```python
from build123d import *

# Parameters (mm, degrees)
ESQUISSE1_W             = 12
ESQUISSE1_H             = 60
MAIN_DEPTH              = 49.95
ESQUISSE2_R             = 1.25
HOLESFIXFORLCD_DEPTH    = 13
SKETCH1_W               = 98
SKETCH1_H               = 40.5
LCDWINDOWHOLE_DEPTH     = 13
SKETCH6_W               = 2.9
SKETCH6_H               = 2
MAKERBEAMRAIL_DEPTH     = 60
SKETCH7_W               = 50
SKETCH7_H               = 9.75
LCDPINSHOLES_DEPTH      = 6
SKETCH8_W               = 8
SKETCH8_H               = 40.5
REINFORCEMENT_DEPTH     = 2.5
REINFORCEMENT_2_DEPTH   = 2.5
SKETCH12_W              = 2.5
SKETCH12_H              = 69
WINDOWPLASTICHOLE_DEPTH = 104.9
SKETCH13_W              = 2.9
SKETCH13_H              = 1
MAKERBEAMRAILUP_DEPTH   = 103.9
BOSS_EXTRUDE2_DEPTH     = 12
SKETCH15_R              = 1.5
CUT_EXTRUDE4_DEPTH      = 7
BOSS_EXTRUDE3_DEPTH     = 10
SKETCH17_R              = 1.5
CUT_EXTRUDE5_DEPTH      = 114.9


with BuildPart() as part:
    # Esquisse1 → Main (new body, symmetric)
    with BuildSketch(Plane.XY):
        with Locations((6, 30)):
            Rectangle(ESQUISSE1_W, ESQUISSE1_H)
    extrude(amount=MAIN_DEPTH, both=True)

    # Esquisse2 → HolesFixForLCD (cut, through all)
    with BuildSketch(Plane(origin=(12, 0, 0), x_dir=(0, 0, -1), z_dir=(1, 0, 0))):
        with Locations((46.4, 2.5)):
            Circle(ESQUISSE2_R)
        with Locations((-46.4, 2.5)):
            Circle(ESQUISSE2_R)
        with Locations((46.4, 57.1)):
            Circle(ESQUISSE2_R)
        with Locations((-46.4, 57.1)):
            Circle(ESQUISSE2_R)
    extrude(amount=-HOLESFIXFORLCD_DEPTH, mode=Mode.SUBTRACT)

    # Sketch1 → LCDWindowHole (cut, through all)
    with BuildSketch(Plane(origin=(12, 0, 0), x_dir=(0, 0, -1), z_dir=(1, 0, 0))):
        with Locations((0, 30)):
            Rectangle(SKETCH1_W, SKETCH1_H)
    extrude(amount=-LCDWINDOWHOLE_DEPTH, mode=Mode.SUBTRACT)

    # Sketch6 → MakerBeamRail (add)
    with BuildSketch(Plane(origin=(0, 60, 0), x_dir=(1, 0, 0), z_dir=(0, 1, 0))):
        with Locations((5, 50.95)):
            Rectangle(SKETCH6_W, SKETCH6_H)
        with Locations((5, -50.95)):
            Rectangle(SKETCH6_W, SKETCH6_H)
    extrude(amount=-MAKERBEAMRAIL_DEPTH)

    # Sketch7 → LCDPinsHoles (cut)
    with BuildSketch(Plane(origin=(12, 0, 0), x_dir=(0, 0, -1), z_dir=(1, 0, 0))):
        with Locations((16.95, 55.125)):
            Rectangle(SKETCH7_W, SKETCH7_H)
    extrude(amount=-LCDPINSHOLES_DEPTH, mode=Mode.SUBTRACT)


with BuildPart() as body_2:
    # Sketch8 → Reinforcement (new body)
    with BuildSketch(Plane.ZY):
        with Locations((-45, 30)):
            Rectangle(SKETCH8_W, SKETCH8_H)
    extrude(amount=-REINFORCEMENT_DEPTH)


with BuildPart() as body_3:
    # Sketch8 → Reinforcement 2 (new body)
    with BuildSketch(Plane.ZY):
        with Locations((45, 30)):
            Rectangle(SKETCH8_W, SKETCH8_H)
    extrude(amount=-REINFORCEMENT_2_DEPTH)


with BuildPart() as windowplastichole_tool:
    # Sketch12 → WindowPlasticHole (new body, through all)
    with BuildSketch(Plane.XY.offset(51.95)):
        with Locations((1.25, 34.5)):
            Rectangle(SKETCH12_W, SKETCH12_H)
    extrude(amount=-WINDOWPLASTICHOLE_DEPTH)


with BuildPart() as part_1:
    add(part.part)

    # WindowPlasticHole: cut by windowplastichole_tool
    add(windowplastichole_tool.part, mode=Mode.SUBTRACT)

    # Sketch13 → MakerBeamRailUp (add)
    with BuildSketch(Plane.XY.offset(51.95)):
        with Locations((5, 60.5)):
            Rectangle(SKETCH13_W, SKETCH13_H)
    extrude(amount=-MAKERBEAMRAILUP_DEPTH)

    # Sketch14 → Boss-Extrude2 (add)
    with BuildSketch(Plane(origin=(0, 0, -49.95), x_dir=(-1, 0, 0), z_dir=(0, 0, -1))):
        Polygon((-12, 60), (-6.45, 60), (-6.45, 61), (-2.5, 61), (-2.5, 55), (-12, 55), align=None)
    extrude(amount=BOSS_EXTRUDE2_DEPTH)

    # Sketch15 → Cut-Extrude4 (cut, through all)
    with BuildSketch(Plane.XZ.offset(-55)):
        with Locations((5, -56.95)):
            Circle(SKETCH15_R)
    extrude(amount=-CUT_EXTRUDE4_DEPTH, mode=Mode.SUBTRACT)

    # Sketch16 → Boss-Extrude3 (add)
    with BuildSketch(Plane(origin=(0, 0, 0), x_dir=(-1, 0, 0), z_dir=(0, -1, 0))):
        Polygon((-2.5, -49.95), (-3.55, -49.95), (-3.55, -51.95), (-10, -51.95), (-10, -41.95), (-2.5, -41.95), align=None)
    extrude(amount=BOSS_EXTRUDE3_DEPTH)

    # Sketch17 → Cut-Extrude5 (cut, through all)
    with BuildSketch(Plane.XY.offset(51.95)):
        with Locations((5, -5)):
            Circle(SKETCH17_R)
    extrude(amount=-CUT_EXTRUDE5_DEPTH, mode=Mode.SUBTRACT)


with BuildPart() as body_2_1:
    add(body_2.part)

    # WindowPlasticHole: cut by windowplastichole_tool
    add(windowplastichole_tool.part, mode=Mode.SUBTRACT)


with BuildPart() as body_3_1:
    add(body_3.part)

    # WindowPlasticHole: cut by windowplastichole_tool
    add(windowplastichole_tool.part, mode=Mode.SUBTRACT)


solid = part_1.part
```
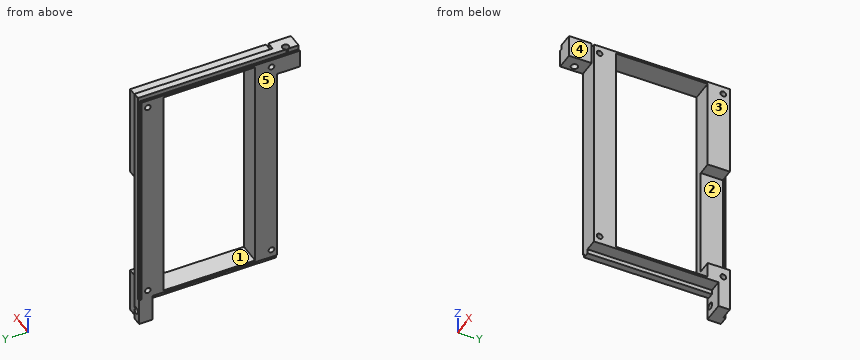
Check sheet for the modelled part. Datum: model origin and axes. Units: mm. Face numbers are marked on the shaded views. A direction names the side the tool comes from. Coordinates: 2 decimals unless noted, no trailing zeros. Loops run counter-clockwise (first coordinate to the right, second up) from the corner with the lowest first, then second, coordinate; pieces in that order, holes last.
1) Sectioned sample at A-A (y = 57.1). Record the boundary of the cut face in (x, z).
2) Material ranges on probe 1 along Y at (x, z) = (6.5, -46.4); probe 2 along Y at (x, z) = (5.25, 46.4); probe 3 along Y at (x, z) = (3.5, -17), recorded low to high.
3) Access from +Z, -Z, +X, -X, +Y, -Y to the whole of each face (thin tool, end or side, straight path). Record for the marked faces 4 and 5.
4) Gauge pin test, flat ends, axial feed: pin 1 (1 mm diameter, centred on x = 9, y = 24.5, fed in from +Z); pin 2 (3 mm diameter, centred on x = 8.5, y = 33.5, fed in from -Z); pin 3 (5 mm diameter, centred on y = 55, z = -6, fed in from +X). Record the tip position at first contact, or that the pin passes through.
5) Sectioned sample at B-B (z = 22.5). Record the boundary of the cut face in (x, y), and give its area (3 significant figures).
6) Sectioned sample at C-C (y = 48.5). Record the boundary of the cut face in (x, z), and give its area (4 significant figures).
7) Sectioned sample at D-D (z = 46.4). Record the boundary of the cut face in (x, y), and give its area (3 significant figures).
8) Release check for a two-part mould opening along Y. For the marked faces 1, 2 and 3 record: released by +Y, released by -Y, zero draft, split by the parting line, or undercut.
Check sheet entries:
1. outline: (2.5, -61.95) - (12, -61.95) - (12, -47.65) - (2.5, -47.65) - close; (2.5, -45.15) - (12, -45.15) - (12, -41.95) - (6, -41.95) - (6, 8.05) - (12, 8.05) - (12, 45.15) - (2.5, 45.15) - close; (2.5, 47.65) - (12, 47.65) - (12, 49.95) - (6.45, 49.95) - (6.45, 51.95) - (3.55, 51.95) - (3.55, 49.95) - (2.5, 49.95) - close; hole circle Ø3 at (5, -56.95)
2. probe 1: y = 0 to 1.25, 3.75 to 9.75, 50.25 to 55.85, 58.35 to 60
2. probe 2: y = -10 to -6.48, -3.52 to 1.25, 3.75 to 9.75, 50.25 to 55.85, 58.35 to 61
2. probe 3: y = 0 to 9.75, 50.25 to 60
3. face 4: +Z, -Z, +X, -Y
3. face 5: +Z, -Z, -X, +Y, -Y
4. pin 1: stops at z = 49.95
4. pin 2: stops at z = -49.95
4. pin 3: stops at x = 6
5. outline: (2.5, 0) - (12, 0) - (12, 9.75) - (2.5, 9.75) - close; (2.5, 50.25) - (12, 50.25) - (12, 60) - (6.45, 60) - (6.45, 61) - (3.55, 61) - (3.55, 60) - (2.5, 60) - close
5. area: 188 mm2
6. outline: (2.5, -49.95) - (3.55, -49.95) - (3.55, -51.95) - (6.45, -51.95) - (6.45, -49.95) - (12, -49.95) - (12, -49) - (2.5, -49) - close; (2.5, 49) - (12, 49) - (12, 49.95) - (6.45, 49.95) - (6.45, 51.95) - (3.55, 51.95) - (3.55, 49.95) - (2.5, 49.95) - close
6. area: 29.65 mm2
7. outline: (2.5, -10) - (10, -10) - (10, 0) - (12, 0) - (12, 1.25) - (2.5, 1.25) - close; (2.5, 3.75) - (12, 3.75) - (12, 9.75) - (2.5, 9.75) - close; (2.5, 50.25) - (12, 50.25) - (12, 55.85) - (2.5, 55.85) - close; (2.5, 58.35) - (12, 58.35) - (12, 60) - (6.45, 60) - (6.45, 61) - (3.55, 61) - (3.55, 60) - (2.5, 60) - close; hole circle Ø3 at (5, -5)
7. area: 209 mm2
8. face 1: undercut
8. face 2: undercut
8. face 3: zero draft
